from build123d import *

# Parameters (mm, degrees)
ESQUISSE1_R             = 7
BASE_EXTRUSION_DEPTH    = 9
BASE_EXTRUSION_DRAFT    = -12.5
ENL_V_MAT_EXTRU_2_DEPTH = 14.37908816


with BuildPart() as part:
    # Esquisse1 → Base-Extrusion (with draft: the straight prism first)
    with BuildSketch(Plane.XY):
        Circle(ESQUISSE1_R)
    extrude(amount=-BASE_EXTRUSION_DEPTH)
    # Base-Extrusion: the draft: its side faces are tilted about the plane it starts from
    base_extrusion_sides = [part.faces().sort_by_distance(p)[0] for p in [
        (-7, 0, -4.5),
    ]]
    draft(base_extrusion_sides, Plane.XY, BASE_EXTRUSION_DRAFT)

    # Esquisse5 → Enlèv. mat.-Extru.2 (cut, through all)
    with BuildSketch(Plane.XY):
        with BuildLine():
            Line((-0.5, 7.599649669), (0.5, 7.599649669))
            Line((0.5, 7.599649669), (0.5, 3.968626967))
            ThreePointArc((0.5, 3.968626967), (0, -4), (-0.5, 3.968626967))
            Line((-0.5, 3.968626967), (-0.5, 7.599649669))
        make_face()
    extrude(amount=-ENL_V_MAT_EXTRU_2_DEPTH, mode=Mode.SUBTRACT)


solid = part.part
Check sheet for the modelled part. Datum: model origin and axes. Units: mm. A direction names the side the tool comes from. Give positions to 0.01 mm unless a question says otherwise; leave off trailing zeros. Write each loop counter-clockwise with the first axis right and the second up, starting at its lowest first coordinate (ties: lowest second). Pieces come first, ordered by that corner, then holes. Notation, with made-up numbers: (38.25, -31.75) -> (57.25, -31.75) arc R32 ccw to (57.25, -1.75) -> close; hole circle Ø11 at (-9, 8). An arc over 180 degrees is marked (long way). Use one line per item in the form item = value. Start each with the question number.
1. Section check B-B (z = -0.75). Record the cut outline in (x, y), and give its area (3 significant figures).
2. Section check A-A (x = 0). Record the cut outline in (y, z).
3. Go/stop test with flat-tipped pins: P1, Ø5, axis at x = -5.5, z = -8, coming from the +Y side; P2, Ø1, axis at y = 2, z = -5.5, coming from the -X side; P3, Ø4, axis at y = 5, z = -2.5, coming from the +X side; P4, Ø6.5, axis at x = 0, y = 0, coming from the -Z side. Record where each tip stops, or that it passes through.
4. Access from +Z, -Z, +X, -X, +Y, -Y to the whole of each face (thin tool, end or side, straight path). Record for faces 1 (the cylindrical face through (0, -4, -4)), 2 (the flat face through (-0.5, 5, -3)).
5. Thickness scan on line 1 along Y through (x, z) = (-2.5, -8.5); line 2 along X through (y, z) = (0, -4.25); line 3 along Y through (x, z) = (-3, -6.5). Record the ranges inside material, lowest first. Write a range as from..to.
6. Mould release check, pull along X, two halves, no side actions. Record for faces 3 (the flat face through (0.5, 5, -3)), 4 (the flat face through (3, -3, 0)): pulls with the +X half, pulls with the -X half, needs draft (parallel to the pull), parting line crosses it, or undercut.
Conclusion:
q1.outline = (-0.5, 3.97) -> (-0.5, 6.82) arc R6.83 ccw (long way) to (0.5, 6.82) -> (0.5, 3.97) arc R4 cw (long way) to start
q1.area = 93.6 mm²
q2.outline = (-7, 0) -> (-5, -9) -> (-4, -9) -> (-4, 0) -> close
q3.P1 = 4.41
q3.P2 = -5.62
q3.P3 = 5.82
q3.P4 = through
q4.face_1 = +Z, -Z
q4.face_2 = +Z, -Z, +Y
q5.line_1 = -4.46..-3.12, 3.12..4.46
q5.line_2 = -6.06..-4, 4..6.06
q5.line_3 = -4.68..-2.65, 2.65..4.68
q6.face_3 = undercut
q6.face_4 = needs draft
